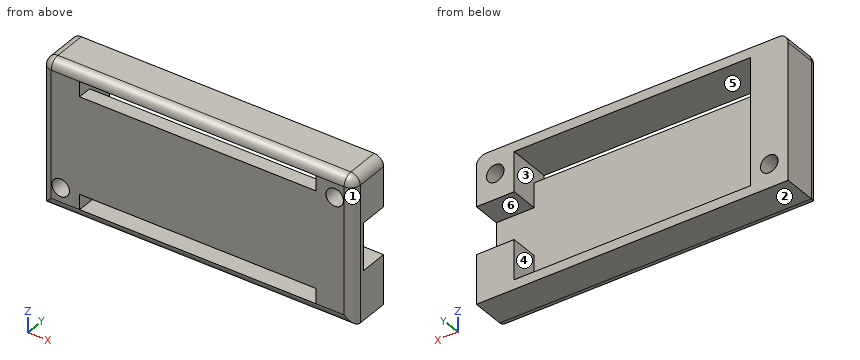
```python
from build123d import *

# Parameters (mm, degrees)
SKETCH1_W           = 66
SKETCH1_H           = 30.8
SKETCH1_W_2         = 50
SKETCH1_H_2         = 3.2
BOSS_EXTRUDE1_DEPTH = 3
SKETCH2_W           = 66
SKETCH2_H           = 30.8
SKETCH2_W_2         = 50
SKETCH2_H_2         = 26.8
BOSS_EXTRUDE2_DEPTH = 6
SKETCH3_R           = 1.85
CUT_EXTRUDE1_DEPTH  = 74.386919815
FILLET1_R           = 2
SKETCH4_W           = 8
SKETCH4_H           = 10
CUT_EXTRUDE2_DEPTH  = 6


with BuildPart() as part:
    # Sketch1 → Boss-Extrude1 (new body)
    with BuildSketch(Plane(origin=(0, 0, 0), x_dir=(1, 0, 0), z_dir=(0, 1, 0))):
        with Locations((33, 15.4)):
            Rectangle(SKETCH1_W, SKETCH1_H)
        with Locations((33, 27.2)):
            Rectangle(SKETCH1_W_2, SKETCH1_H_2, mode=Mode.SUBTRACT)
        with Locations((33, 3.6)):
            Rectangle(SKETCH1_W_2, SKETCH1_H_2, mode=Mode.SUBTRACT)
    extrude(amount=BOSS_EXTRUDE1_DEPTH)

    # Sketch2 → Boss-Extrude2 (add)
    with BuildSketch(Plane(origin=(0, 3, 0), x_dir=(1, 0, 0), z_dir=(0, 1, 0))):
        with Locations((33, 15.4)):
            Rectangle(SKETCH2_W, SKETCH2_H)
        with Locations((33, 15.4)):
            Rectangle(SKETCH2_W_2, SKETCH2_H_2, mode=Mode.SUBTRACT)
    extrude(amount=BOSS_EXTRUDE2_DEPTH)

    # Sketch3 → Cut-Extrude1 (cut, through all)
    with BuildSketch(Plane(origin=(0, 9, 0), x_dir=(1, 0, 0), z_dir=(0, 1, 0))):
        with Locations(Location((62, 5, 0), (0, 0, 270))):
            Circle(SKETCH3_R)
        with Locations(Location((4, 25.8, 0), (0, 0, 270))):
            Circle(SKETCH3_R)
    extrude(amount=-CUT_EXTRUDE1_DEPTH, mode=Mode.SUBTRACT)

    # Fillet1
    fillet1_edges = [part.edges().sort_by_distance(p)[0] for p in [
        (33, 0, -30.8),
        (66, 0, -15.4),
        (33, 0, 0),
        (0, 0, -15.4),
        (66, 4.5, 0),
        (0, 4.5, 0),
    ]]
    fillet(fillet1_edges, radius=FILLET1_R - 0.0001)  # a hair under: the kernel refuses the full size

    # Sketch4 → Cut-Extrude2 (cut)
    with BuildSketch(Plane(origin=(0, 9, 0), x_dir=(1, 0, 0), z_dir=(0, 1, 0))):
        with Locations((62, 15.4)):
            Rectangle(SKETCH4_W, SKETCH4_H)
    extrude(amount=-CUT_EXTRUDE2_DEPTH, mode=Mode.SUBTRACT)


solid = part.part
```
Design review of the part built by this model. Coordinates are the model's own, in mm. Face numbers are marked on the shaded views. A direction names the side the tool comes from. Give positions to 0.01 mm unless a question says otherwise; leave off trailing zeros. Write each loop counter-clockwise with the first axis right and the second up, starting at its lowest first coordinate (ties: lowest second). Pieces come first, ordered by that corner, then holes. Notation, with made-up numbers: (10.25, 33) -> (54.25, 33) arc R30 cw to (54.25, 61) -> close; hole circle Ø2 at (-4.5, 62.25). An arc over 180 degrees is marked (long way). Answer in a Markdown table with one row per item.
(1) Consider section D-D (y = 1). State the section outline as (x, z) points.
Results:
| item | result |
|---|---|
| outline | (0.27, -30.53) -> (65.73, -30.53) -> (65.73, -2) arc R1.73 ccw to (64, -0.27) -> (2, -0.27) arc R1.73 ccw to (0.27, -2) -> close; hole circle Ø3.7 at (4, -25.8); hole (8, -28.8) -> (58, -28.8) -> (58, -25.6) -> (8, -25.6) -> close; hole (8, -5.2) -> (58, -5.2) -> (58, -2) -> (8, -2) -> close; hole circle Ø3.7 at (62, -5) |
(2) To check wall thickness, follow probe 1 along X at (y, z) = (3, -5); probe 2 along X at (y, z) = (7, -25.8); probe 3 along Z at (x, y) = (13, 4.25). State the ranges of each line that lie inside material, in increasing order.
Results:
| item | result |
|---|---|
| probe 1 | 0 to 8, 58 to 60.15, 63.85 to 66 |
| probe 2 | 0 to 2.15, 5.85 to 8, 58 to 66 |
| probe 3 | -30.8 to -28.8, -2 to 0 |
(3) Clearance check with flat-ended pins moving along their axes: pin 1 (10 mm diameter, centred on x = 37.5, z = -13.5, fed in from +Y); pin 2 (3 mm diameter, centred on x = 4, z = -25.8, fed in from -Y). State where each tip first meets the part, or that it passes through.
Results:
| item | result |
|---|---|
| pin 1 | y = 3 |
| pin 2 | through |
(4) Mouldability with a two-part tool opening along X and no side actions: class the marked faces 1, 2 and 3 as +X half, -X half, draft (parallel to the pull), parting line (faces both ways), or undercut.
Results:
| item | result |
|---|---|
| face 1 | +X half |
| face 2 | draft |
| face 3 | undercut |
(5) Consider section A-A (x = 62). State the section outline as (y, z) points.
Results:
| item | result |
|---|---|
| outline | (0, -28.8) arc R2 ccw to (2, -30.8) -> (9, -30.8) -> (9, -20.4) -> (3, -20.4) -> (3, -10.4) -> (9, -10.4) -> (9, -6.85) -> (0, -6.85) -> close; (0, -3.15) -> (9, -3.15) -> (9, 0) -> (2, 0) arc R2 ccw to (0, -2) -> close |
(6) Consider section B-B (y = 7). State the section outline as (x, z) points.
Results:
| item | result |
|---|---|
| outline | (0, -30.8) -> (66, -30.8) -> (66, -20.4) -> (58, -20.4) -> (58, -28.8) -> (8, -28.8) -> (8, -2) -> (58, -2) -> (58, -10.4) -> (66, -10.4) -> (66, -2) arc R2 ccw to (64, 0) -> (2, 0) arc R2 ccw to (0, -2) -> close; hole circle Ø3.7 at (4, -25.8); hole circle Ø3.7 at (62, -5) |
(7) For the marked faces 4, 5 and 6, list the 3-axis set-ups (+Z, -Z, +X, -X, +Y, -Y) from which the entire face can be reached by the end or side of a thin tool; tool diameter is ignored.
Results:
| item | result |
|---|---|
| face 4 | +Y |
| face 5 | +Y, -Y |
| face 6 | +X, +Y |
(8) Consider section C-C (x = 33.5). Count the separate pieces of the cut face and the enclosed holes in it, then the cut area to 3 significant figures.
Results:
| item | result |
|---|---|
| separate pieces | 3 |
| enclosed holes | 0 |
| area | 95.5 mm2 |
